```python
from build123d import *

# Parameters (mm, degrees)
BOSS_EXTRUDE1_DEPTH = 10
CUT_EXTRUDE1_DEPTH  = 10


with BuildPart() as part:
    # Sketch1 → Boss-Extrude1 (new body)
    with BuildSketch(Plane.XY):
        with BuildLine():
            Line((-50, 60), (50, 60))
            ThreePointArc((50, 60), (57.071067812, 57.071067812), (60, 50))
            Line((60, 50), (60, -50))
            ThreePointArc((60, -50), (57.071067812, -57.071067812), (50, -60))
            Line((50, -60), (-50, -60))
            ThreePointArc((-50, -60), (-57.071067812, -57.071067812), (-60, -50))
            Line((-60, -50), (-60, 50))
            ThreePointArc((-60, 50), (-57.071067812, 57.071067812), (-50, 60))
        make_face()
    extrude(amount=BOSS_EXTRUDE1_DEPTH)

    # Sketch2 → Cut-Extrude1 (cut)
    with BuildSketch(Plane.XY.offset(10)):
        with BuildLine():
            Line((0.576923077, 24.358974359), (-16.474358974, 24.358974359))
            add(Edge.make_bspline(
                [(-16.474358974, 24.358974359), (-16.353970438, 25.211307119), (-16.117956688, 26.882249036), (-15.553207348, 29.301356677), (-14.877706194, 31.596045832), (-14.034377515, 33.75904969), (-13.045290174, 35.794221276), (-11.920502083, 37.708544306), (-10.647853859, 39.493802146), (-9.672355516, 40.569248555), (-9.185697115, 41.105769231)],
                knots=[0, 0, 0, 0, 1.111473889, 2.178970933, 3.205615836, 4.199322666, 5.174200091, 6.12565194, 7.064921805, 8, 8, 8, 8], degree=3))
            add(Edge.make_bspline(
                [(-9.185697115, 41.105769231), (-8.483756858, 41.813669386), (-7.10030638, 43.208866194), (-4.788398372, 44.995959193), (-2.365091827, 46.542566651), (0.218213736, 47.768728226), (2.92132013, 48.761163974), (5.765723399, 49.427785309), (8.739800279, 49.87009445), (10.769233604, 49.913663441), (11.804887821, 49.935897436)],
                knots=[0, 0, 0, 0, 1.01925491, 2.00884431, 2.983262333, 3.955970413, 4.92937149, 5.924503185, 6.940838805, 8, 8, 8, 8], degree=3))
            add(Edge.make_bspline(
                [(11.804887821, 49.935897436), (12.725637707, 49.914160335), (14.535646445, 49.871429576), (17.19590386, 49.528410226), (19.732236676, 48.926792485), (22.171454673, 48.140190789), (24.477684901, 47.069887718), (26.701828098, 45.82749366), (28.781741625, 44.303645718), (30.722292085, 42.581850898), (32.505057791, 40.719561249), (34.048940704, 38.728926766), (35.376244548, 36.663121884), (36.469767354, 34.504983674), (37.31053779, 32.250860305), (37.894057408, 29.913773543), (38.275985165, 27.498880346), (38.31403515, 25.857509967), (38.333333333, 25.025040064)],
                knots=[0, 0, 0, 0, 1.091422571, 2.145516843, 3.172569842, 4.178562979, 5.178154469, 6.181868002, 7.194278174, 8.227918432, 9.254613415, 10.245994977, 11.209837596, 12.161663635, 13.10878368, 14.055455738, 15.013766427, 16, 16, 16, 16], degree=3))
            add(Edge.make_bspline(
                [(38.333333333, 25.025040064), (38.293732308, 23.994095409), (38.215770063, 21.964482346), (37.576033403, 18.993992832), (36.574671568, 16.153674752), (35.128107, 13.483268429), (33.319532856, 10.990041205), (31.100472953, 8.757349154), (28.534131878, 6.750186691), (26.607545449, 5.671537337), (25.62099359, 5.119190705)],
                knots=[0, 0, 0, 0, 0.992805628, 1.954529043, 2.915727527, 3.886831945, 4.871318353, 5.87440735, 6.911542536, 8, 8, 8, 8], degree=3))
            add(Edge.make_bspline(
                [(25.62099359, 5.119190705), (26.298147652, 4.896866769), (27.628725011, 4.460010206), (29.51998074, 3.599626149), (31.31834883, 2.659368988), (32.99286203, 1.567038026), (34.560175394, 0.366802286), (36.010734394, -0.951598279), (37.353205786, -2.385288944), (38.565674269, -3.942154462), (39.641787421, -5.5972958), (40.607326451, -7.312480175), (41.402018895, -9.113718663), (42.07522233, -10.980439908), (42.587761098, -12.929421022), (42.94863419, -14.953109858), (43.157227694, -17.046890251), (43.189041761, -18.465425199), (43.205128205, -19.182692308)],
                knots=[0, 0, 0, 0, 1.059543567, 2.081955587, 3.086750234, 4.076226789, 5.052108497, 6.020845489, 6.989030705, 7.970690546, 8.952259656, 9.923888338, 10.895517021, 11.877585046, 12.873342345, 13.889638361, 14.932918083, 16, 16, 16, 16], degree=3))
            add(Edge.make_bspline(
                [(43.205128205, -19.182692308), (43.17251882, -20.236783738), (43.108219755, -22.315237362), (42.699436391, -25.376586846), (41.938355422, -28.295311592), (40.937111249, -31.104995931), (39.601560188, -33.769367864), (38.029841121, -36.34957109), (36.097882591, -38.756124872), (33.950842418, -41.052652256), (31.566429135, -43.140552122), (28.981337229, -44.950667352), (26.252410658, -46.504068279), (23.362384275, -47.765163409), (20.312262141, -48.736350893), (17.108842711, -49.438369972), (13.738666093, -49.86787686), (11.438256871, -49.912902514), (10.263421474, -49.935897436)],
                knots=[0, 0, 0, 0, 1.005138573, 1.981928558, 2.936866704, 3.876260664, 4.820238198, 5.773547, 6.751179199, 7.756627054, 8.768222608, 9.766606018, 10.760583154, 11.757261445, 12.767156078, 13.807575856, 14.880313354, 16, 16, 16, 16], degree=3))
            add(Edge.make_bspline(
                [(10.263421474, -49.935897436), (9.152046138, -49.911653178), (6.978898733, -49.86424674), (3.800215835, -49.453919993), (0.779178625, -48.792029652), (-2.09192263, -47.859040331), (-4.801979884, -46.649112625), (-7.375568975, -45.208360206), (-9.761334505, -43.453683826), (-11.985858603, -41.464292892), (-13.999794607, -39.232309222), (-15.799779124, -36.809435607), (-17.34612218, -34.186458852), (-18.645165347, -31.374585409), (-19.686753045, -28.368882405), (-20.508354364, -25.175462089), (-21.082256332, -21.788085508), (-21.25703938, -19.457498358), (-21.346153846, -18.269230769)],
                knots=[0, 0, 0, 0, 1.066544725, 2.085487077, 3.070979577, 4.031932826, 4.977951092, 5.916076795, 6.857635327, 7.814973522, 8.776389752, 9.738577119, 10.707772778, 11.69409279, 12.707140348, 13.757286496, 14.856535458, 16, 16, 16, 16], degree=3))
            Line((-21.346153846, -18.269230769), (-4.294871795, -18.269230769))
            add(Edge.make_bspline(
                [(-4.294871795, -18.269230769), (-4.186819599, -18.866707312), (-3.97635961, -20.030449564), (-3.56587031, -21.715289641), (-3.030945483, -23.270501097), (-2.412439293, -24.709906604), (-1.744359491, -26.052405056), (-0.937159331, -27.248414671), (-0.049986198, -28.330412012), (1.2302111, -29.616702375), (3.060341313, -30.938312023), (5.531623414, -32.086853681), (8.280690724, -32.7600402), (10.202562942, -32.842166887), (11.195913462, -32.884615385)],
                knots=[0, 0, 0, 0, 0.928156231, 1.807827665, 2.648129825, 3.438902246, 4.202261636, 4.936546065, 5.639352463, 6.338805438, 7.70633318, 9.064371875, 10.482673459, 12, 12, 12, 12], degree=3))
            add(Edge.make_bspline(
                [(11.195913462, -32.884615385), (11.723020359, -32.875576377), (12.755504848, -32.857870983), (14.272070822, -32.661630398), (15.716813447, -32.338422007), (17.092423634, -31.899193782), (18.407658596, -31.34859374), (19.637389454, -30.638627935), (20.8066812, -29.813191335), (21.902822566, -28.885181468), (22.915679777, -27.873982913), (23.758436542, -26.754252311), (24.528655243, -25.616405886), (25.098314545, -24.386001717), (25.597458818, -23.129248692), (25.902960612, -21.800530617), (26.133636405, -20.427720421), (26.147042356, -19.488229388), (26.153846154, -19.011418269)],
                knots=[0, 0, 0, 0, 1.110435564, 2.175094844, 3.216326037, 4.226890168, 5.215276772, 6.21526065, 7.213097102, 8.228249917, 9.239874822, 10.221364777, 11.178138315, 12.128914389, 13.072518965, 14.022636769, 14.996447288, 16, 16, 16, 16], degree=3))
            add(Edge.make_bspline(
                [(26.153846154, -19.011418269), (26.135783345, -18.489944075), (26.099824432, -17.451808443), (25.806036347, -15.936867778), (25.342082867, -14.479616956), (24.697594812, -13.086509368), (23.836952841, -11.762679732), (22.821404918, -10.481568019), (21.570942657, -9.309853806), (20.199018093, -8.151649816), (18.608124558, -7.142045251), (16.8757408, -6.210328579), (14.956337088, -5.468969755), (12.896767777, -4.806799007), (10.658074191, -4.323159778), (8.254157787, -3.971990559), (5.688896433, -3.710599501), (3.920628445, -3.673098649), (3.012820513, -3.653846154)],
                knots=[0, 0, 0, 0, 0.809814727, 1.612155564, 2.388397, 3.182215007, 3.988903953, 4.837162975, 5.715530372, 6.646997145, 7.623086902, 8.637258368, 9.698941581, 10.815059213, 11.996518529, 13.252603015, 14.589518788, 16, 16, 16, 16], degree=3))
            Line((3.012820513, -3.653846154), (3.012820513, 12.179487179))
            add(Edge.make_bspline(
                [(3.012820513, 12.179487179), (4.143095378, 12.275745003), (6.257615816, 12.455824329), (9.192683563, 12.876946094), (11.663632261, 13.439844668), (13.729851196, 14.118951328), (15.445507012, 14.991101207), (16.944294459, 15.953916158), (18.235121106, 17.072085016), (19.326042778, 18.312264133), (20.198746175, 19.644100211), (20.816394798, 21.04689257), (21.22425768, 22.477237082), (21.262902657, 23.455549618), (21.282051282, 23.940304487)],
                knots=[0, 0, 0, 0, 1.70044513, 3.18119609, 4.440695891, 5.496282586, 6.431922213, 7.318171381, 8.16090191, 8.983045123, 9.787564368, 10.536848927, 11.275007137, 12, 12, 12, 12], degree=3))
            add(Edge.make_bspline(
                [(21.282051282, 23.940304487), (21.249014421, 24.558799065), (21.184533463, 25.76596954), (20.683739411, 27.493684792), (19.814417678, 29.033799739), (18.648809879, 30.383073548), (17.228476249, 31.510088157), (15.563596248, 32.328281547), (13.690297868, 32.809006698), (12.37233152, 32.858841698), (11.690705128, 32.884615385)],
                knots=[0, 0, 0, 0, 1.009664648, 1.970651636, 2.907870547, 3.878035693, 4.867062054, 5.849714035, 6.887914197, 8, 8, 8, 8], degree=3))
            add(Edge.make_bspline(
                [(11.690705128, 32.884615385), (11.072887442, 32.854205145), (9.846947924, 32.793861915), (8.05425741, 32.343476035), (6.351798685, 31.585307457), (4.774824861, 30.539837669), (3.346099876, 29.284272772), (2.173528872, 27.797316766), (1.198239906, 26.168055763), (0.784840597, 24.964365524), (0.576923077, 24.358974359)],
                knots=[0, 0, 0, 0, 0.98818071, 1.960853194, 2.938124878, 3.957524365, 4.978590984, 5.968022688, 6.978025184, 8, 8, 8, 8], degree=3))
        make_face()
    extrude(amount=-CUT_EXTRUDE1_DEPTH, mode=Mode.SUBTRACT)


solid = part.part
```
Read the model definition and answer for the solid it produces. Units are mm, in the model's axes. A direction names the side the tool comes from. Coordinates: 2 decimals unless noted, no trailing zeros. Answer as a JSON object with one key per item and string values. Group by question number.
Item 1: Section A-A (x = 28.5) is taken. State how many separate pieces and enclosed holes the cut face has, plus the area to 3 significant figures.
Item 2: Consider probe 1 along Y at (x, z) = (30, 0.75); probe 2 along Y at (x, z) = (-9, 9.5); probe 3 along Y at (x, z) = (13, 3). Determine where each line is inside the solid, lowest interval first. Write a range as from..to.
Item 3: The mould has two halves that part along Y. Classify faces 1 (the face through (-13, -18.269, 5)), 2 (the face through (-56.99, -57.15, 4.93)), 3 (the face through (1, 1, 10)): +Y half, -Y half, draft (parallel to the pull), parting line (faces both ways), or undercut.
Item 4: A tool of negligible diameter and unlimited length cuts with its end or side. For faces 4 (the face through (3.013, 4, 5)), 5 (the face through (-57.15, 56.99, 4.93)), from which of +Z, -Z, +X, -X, +Y, -Y can it reach the whole face along a straight path? Write none if from no direction.
Results are:
{
 "1": {"separate pieces": "3", "enclosed holes": "0", "area": "331 mm^2"},
 "2": {"probe 1": "y = -60..-44.22, 3.34..7.92, 43.21..60", "probe 2": "y = -60..-43.99, -18.27..24.36, 41.29..60", "probe 3": "y = -60..-49.85, -32.81..-4.87, 13.89..32.82, 49.9..60"},
 "3": {"face 1": "undercut", "face 2": "-Y half", "face 3": "draft"},
 "4": {"face 4": "+Z, -Z", "face 5": "+Z, -Z, -X, +Y"}
}
